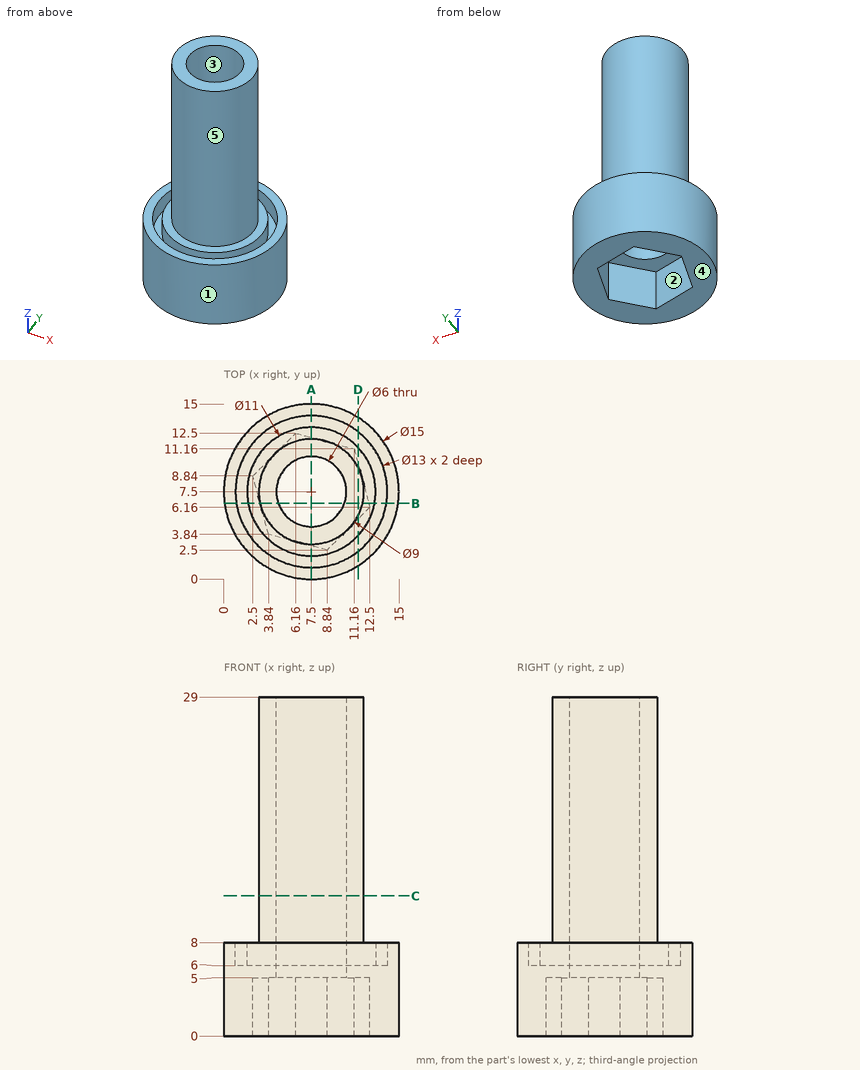
Design review of the part shown in the three views and the two pictorial views. Dimensions are in mm from the part's minimum x, y and z. A direction names the side the tool comes from. Give positions to 0.01 mm unless a question says otherwise; leave off trailing zeros. Loops run counter-clockwise (first coordinate to the right, second up) from the corner with the lowest first, then second, coordinate; pieces in that order, holes last. Notation, with made-up numbers: M 33.25,-22 L 43.25,-22 A13 cw 43.25,-15 Z; hole C 52,-28.5 d1. An arc over 180 degrees is marked long. Answer as a JSON object with one key per item and string values. Group by question number.
Q1. Insertion check: P1, Ø3, axis at x = 12.5, z = 3.5, coming from the -Y side; P2, Ø1.5, axis at y = 6.5, z = 6, coming from the -X side; P3, Ø1.5, axis at y = 11.5, z = 15, coming from the -X side. Each pin has a flat end and moves straight along its axis. Give the tip position at first contact, or say it passes through.
Q2. For probe 1 along Y at (x, z) = (7.5, 7.2); probe 2 along Y at (x, z) = (7.5, 22.5); probe 3 along Z at (x, y) = (10.25, 5.5), list the stretches that pass through material, from the lowest coordinate up. Write a range as [from, to].
Q3. Add section C-C on z = 12. Give the boundary of the cut face in (x, y).
Q4. Add section A-A on x = 7.5. Give the boundary of the cut face in (y, z).
Q5. Add section D-D on x = 11.5. Give the boundary of the cut face in (y, z) (1 decimal), and give its area (3 significant figures).
Q6. Mouldability with a two-part tool opening along X and no side actions: class the marked faces 3, 4 and 5 as +X half, -X half, draft (parallel to the pull), parting line (faces both ways), or undercut.
Q7. Tool access review of the marked faces 1 and 2: name each direction out of +Z, -Z, +X, -X, +Y, -Y from which nothing blocks a thin tool from reaching the whole face with its end or side.
Q8. Add section B-B on y = 6.5. Give the boundary of the cut face in (x, z).
Checked values:
{
 "1": {"P1": "y = 0.87", "P2": "x = 0", "P3": "x = 4.39"},
 "2": {"probe 1": "[0, 1], [2, 4.5], [10.5, 13], [14, 15]", "probe 2": "[3, 4.5], [10.5, 12]", "probe 3": "[5, 29]"},
 "3": {"outline": "C 7.5,7.5 d9; hole C 7.5,7.5 d6"},
 "4": {"outline": "M 0,0 L 2.86,0 L 2.86,5 L 4.5,5 L 4.5,29 L 3,29 L 3,8 L 2,8 L 2,6 L 1,6 L 1,8 L 0,8 Z; M 10.5,5 L 12.14,5 L 12.14,0 L 15,0 L 15,8 L 14,8 L 14,6 L 13,6 L 13,8 L 12,8 L 12,29 L 10.5,29 Z"},
 "5": {"outline": "M 1.2,0 L 5.2,0 L 5.2,5 L 9.9,5 L 9.9,0 L 13.8,0 L 13.8,8 L 12.6,8 L 12.6,6 L 11.3,6 L 11.3,8 L 9.6,8 L 9.6,29 L 5.4,29 L 5.4,8 L 3.7,8 L 3.7,6 L 2.4,6 L 2.4,8 L 1.2,8 Z", "area": "159 mm²"},
 "6": {"face 3": "undercut", "face 4": "draft", "face 5": "parting line"},
 "7": {"face 1": "+Z, -Z", "face 2": "-Z"},
 "8": {"outline": "M 0.07,0 L 3.13,0 L 3.13,5 L 4.67,5 L 4.67,29 L 3.11,29 L 3.11,8 L 2.09,8 L 2.09,6 L 1.08,6 L 1.08,8 L 0.07,8 Z; M 10.33,5 L 12.41,5 L 12.41,0 L 14.93,0 L 14.93,8 L 13.92,8 L 13.92,6 L 12.91,6 L 12.91,8 L 11.89,8 L 11.89,29 L 10.33,29 Z"}
}
